Autodesk Inventor part; units mm, degrees
ref_plane "YZ Plane" through (0, 0, 0) normal (1, 0, 0) x (0, 1, 0)
ref_plane "XZ Plane" through (0, 0, 0) normal (0, 1, 0) x (-1, 0, 0)
ref_plane "XY Plane" through (0, 0, 0) normal (0, 0, 1) x (1, 0, 0)
sketch "Sketch2" plane through (0, 0, 0) normal (0, 0, 1) x (1, 0, 0)
  line L0 (0, 31.75) -> (44.45, 31.75)
  line L1 (44.45, 31.75) -> (44.45, 0)
  line L2 (44.45, 0) -> (0, 0)
  line L3 (0, 0) -> (0, 31.75)
  circle A0 centre (22.225, 22.225) radius 0.7937
  circle A1 centre (22.225, 9.525) radius 0.7937
  circle A2 centre (28.575, 15.875) radius 0.7937
  circle A3 centre (15.875, 15.875) radius 0.7937
  line L4 (4.7625, 26.9875) -> (11.1125, 26.9875)
  line L5 (11.1125, 26.9875) -> (11.1125, 4.7625)
  line L6 (11.1125, 4.7625) -> (4.7625, 4.7625)
  line L7 (4.7625, 4.7625) -> (4.7625, 26.9875)
  line L8 (33.3375, 26.9875) -> (39.6875, 26.9875)
  line L9 (39.6875, 26.9875) -> (39.6875, 4.7625)
  line L10 (39.6875, 4.7625) -> (33.3375, 4.7625)
  line L11 (33.3375, 4.7625) -> (33.3375, 26.9875)
  dimension "d9" = 44.45
  dimension "d10" = 31.75
  dimension "d11" = 1.5875
  dimension "d12" = 1.5875
  dimension "d13" = 1.5875
  dimension "d14" = 1.5875
  dimension "d15" = 12.7
  dimension "d16" = 12.7
  dimension "d17" = 15.875
  dimension "d18" = 22.225
  dimension "d21" = 6.35
  dimension "d22" = 6.35
  dimension "d26" = 4.7625
  dimension "d27" = 4.7625
  dimension "d28" = 4.7625
  dimension "d29" = 4.7625
  dimension "d30" = 4.7625
  dimension "d31" = 4.7625
extrude "Extrusion4" add sketch "Sketch2" along normal blind 1.5875
fillet "Fillet2" radius 6.35 4 edges at (0, 31.75, 0.7937) (0, 0, 0.7937) (44.45, 0, 0.7937) (44.45, 31.75, 0.7937)
fillet "Fillet3" radius 1.5875 8 edges at (4.7625, 4.7625, 0.7937) (11.1125, 4.7625, 0.7937) (33.3375, 4.7625, 0.7937) (4.7625, 26.9875, 0.7937) (11.1125, 26.9875, 0.7937) (39.6875, 26.9875, 0.7937) (33.3375, 26.9875, 0.7937) (39.6875, 4.7625, 0.7937)
sketch "Sketch3" plane through (0, 0, 1.5875) normal (0, 0, 1) x (1, 0, 0)
  line L0 (13.4937, 18.2563) -> (18.2562, 18.2563)
  line L1 (18.2562, 18.2563) -> (18.2562, 13.4938)
  line L2 (18.2562, 13.4938) -> (13.4937, 13.4938)
  line L3 (13.4937, 13.4938) -> (13.4937, 18.2563)
  circle A0 centre (15.875, 15.875) radius 0.7937
  line L4 (19.8437, 24.6063) -> (24.6062, 24.6063)
  line L5 (24.6062, 24.6063) -> (24.6062, 19.8438)
  line L6 (24.6062, 19.8438) -> (19.8437, 19.8438)
  line L7 (19.8437, 19.8438) -> (19.8437, 24.6063)
  line L8 (26.1937, 18.2563) -> (30.9562, 18.2563)
  line L9 (30.9562, 18.2563) -> (30.9562, 13.4938)
  line L10 (30.9562, 13.4938) -> (26.1937, 13.4938)
  line L11 (26.1937, 13.4938) -> (26.1937, 18.2563)
  line L12 (19.8437, 11.9063) -> (24.6062, 11.9063)
  line L13 (24.6062, 11.9063) -> (24.6062, 7.1438)
  line L14 (24.6062, 7.1438) -> (19.8437, 7.1438)
  line L15 (19.8437, 7.1438) -> (19.8437, 11.9063)
  circle A1 centre (22.225, 22.225) radius 0.7937
  circle A2 centre (28.575, 15.875) radius 0.7937
  circle A3 centre (22.225, 9.525) radius 0.7937
  point P0 (0, 0)
  dimension "d36" = 4.7625
  dimension "d37" = 2.3813
  dimension "d38" = 2.3813
  dimension "d39" = 4.7625
  dimension "d41" = 2.3813
  dimension "d42" = 2.3813
  dimension "d43" = 2.3813
  dimension "d44" = 2.3813
  dimension "d45" = 2.3813
  dimension "d46" = 2.3813
extrude "Extrusion6" cut sketch "Sketch3" against normal blind 0.7937
equation "\"d12\" = d11"
equation "\"d13\" = d11"
equation "\"d14\" = d11"
equation "\"d17\" = 0.5 * d10"
equation "\"d18\" = 0.5 * d9"
equation "\"d28\" = d30"
equation "\"d29\" = d31"
equation "\"d37\" = 0.5 * d36"
equation "\"d38\" = 0.5 * d36"
equation "\"d39\" = d36"
equation "\"d41\" = d37"
equation "\"d42\" = d41"
equation "\"d43\" = d37"
equation "\"d44\" = d37"
equation "\"d45\" = d37"
equation "\"d46\" = d37"
properties part number "extender-plate"
Geometry check sheet. Reference: the model listing, model coordinates, mm. A direction names the side the tool comes from. Round coordinates to 2 decimals unless told otherwise and drop trailing zeros. Loops run counter-clockwise (first coordinate to the right, second up) from the corner with the lowest first, then second, coordinate; pieces in that order, holes last.
Item 1: Access from +Z, -Z, +X, -X, +Y, -Y to the whole of each face (thin tool, end or side, straight path). Record for faces 5 (the flat face through (22, 16, 0)), 6 (the cylindrical face through (5.215, 5.24, 0.805)), 7 (the flat face through (22.2, 23.3, 0.794)).
Item 2: Cross-section at B-B on x = 17.5. Record the boundary of the cut face in (y, z).
Item 3: Cross-section at C-C on z = 0.3. Count the separate pieces of the cut face and the enclosed holes in it, then the cut area to 3 significant figures.
Item 4: Cross-section at A-A on y = 13. Record the boundary of the cut face in (x, z), then the cut area to 3 significant figures.
Item 5: Gauge pin test, flat end, axial feed: pin 1 (2 mm diameter, centred on x = 22.225, y = 22.225, fed in from +Z). Record the tip position at first contact, or that the pin passes through.
Item 6: Cross-section at D-D on x = 3.5. Record the boundary of the cut face in (y, z).
Item 7: Thickness scan on line 1 (X direction, y = 6.5, z = 1.05); line 2 (Y direction, x = 27, z = 1.25); line 3 (Y direction, x = 24.5, z = 1.55). Record the ranges inside material, lowest first.
Item 8: Mould release check, pull along Y, two halves, no side actions. Record for faces 1 (the flat face through (0, 16, 1)), 2 (the cylindrical face through (1.91, 29.94, 0.8)), 3 (the flat face through (22, 0, 1)), 4 (the cylindrical face through (39.235, 26.51, 0.805)): pulls with the +Y half, pulls with the -Y half, needs draft (parallel to the pull), parting line crosses it, or undercut.
Answer sheet:
1. face 5: -Z, +X, -X, +Y, -Y
1. face 6: +Z, -Z
1. face 7: +Z
2. outline: (0, 0) - (31.75, 0) - (31.75, 1.59) - (18.26, 1.59) - (18.26, 0.79) - (13.49, 0.79) - (13.49, 1.59) - (0, 1.59) - close
3. separate pieces: 1
3. enclosed holes: 6
3. area: 1,090 mm2
4. outline: (0, 0) - (4.76, 0) - (4.76, 1.59) - (0, 1.59) - close; (11.11, 0) - (33.34, 0) - (33.34, 1.59) - (11.11, 1.59) - close; (39.69, 0) - (44.45, 0) - (44.45, 1.59) - (39.69, 1.59) - close
4. area: 50.4 mm2
5. pin 1: stops at z = 0.79
6. outline: (0.68, 0) - (31.07, 0) - (31.07, 1.59) - (0.68, 1.59) - close
7. line 1: x = 0 to 4.76, 11.11 to 33.34, 39.69 to 44.45
7. line 2: y = 0 to 13.49, 18.26 to 31.75
7. line 3: y = 0 to 7.14, 11.91 to 19.84, 24.61 to 31.75
8. face 1: needs draft
8. face 2: pulls with the +Y half
8. face 3: pulls with the -Y half
8. face 4: undercut
